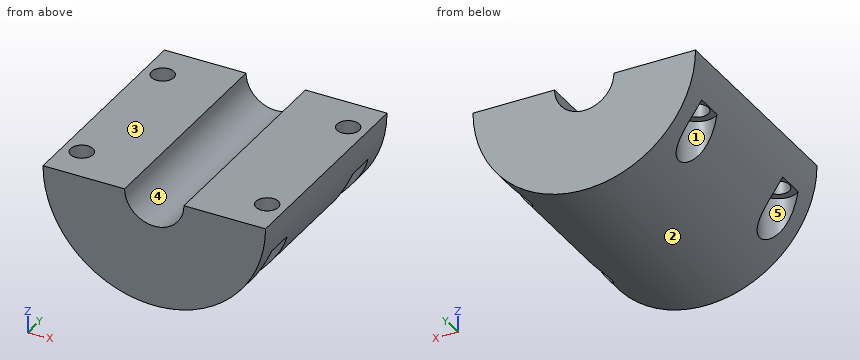
Solid Edge part; units mm, degrees
sketch "Sketch1" plane through (0, 0, 0) normal (0, -1, 0) x (1, 0, 0)
  line L0 (4, 0) -> (15, 0)
  line L1 (-15, 0) -> (-4, 0)
  arc A0 (-4, 0) -> (4, 0) centre (0, 0) ccw
  arc A1 (15, 0) -> (-15, 0) centre (0, 0) cw
extrude "Protrusion1" add sketch "Sketch1" against normal blind 30
sketch "Sketch2" plane through (-9.5, 15, 0) normal (0, 0, 1) x (1, 0, 0)
  circle A0 centre (-3, 10) radius 1.5
  circle A1 centre (22, 10) radius 1.5
  circle A2 centre (22, -10) radius 1.5
  circle A3 centre (-3, -10) radius 1.5
extrude "ExtrudedCutout_1" cut sketch "Sketch2" against normal blind 20
sketch "Sketch3" plane through (9.5, 15, -10) normal (0, 0, 1) x (0, -1, 0)
  circle A0 centre (-10, 3) radius 2.5
  circle A1 centre (10, 3) radius 2.5
  circle A2 centre (-10, -22) radius 2.5
  circle A3 centre (10, -22) radius 2.5
extrude "ExtrudedCutout_2" cut sketch "Sketch3" along normal mid plane 10
For this review, take the finished solid that the model builds, in its own axes (mm). Face numbers are marked on the shaded views. A direction names the side the tool comes from. Round coordinates to 2 decimals unless told otherwise and drop trailing zeros. Loops run counter-clockwise (first coordinate to the right, second up) from the corner with the lowest first, then second, coordinate; pieces in that order, holes last. Notation, with made-up numbers: (15.25, 6) - (63.25, 6) arc R18 ccw to (63.25, 11) - close; hole circle Ø8 at (-17.5, 86.25). An arc over 180 degrees is marked (long way). One line per item, written item: value. Start each with the question number.
Item 1: Take a section at B-B (x = 13.5). Give the boundary of the cut face in (y, z).
Item 2: Take a section at C-C (z = -7.5). Give the boundary of the cut face in (x, y), plus the area to 3 significant figures.
Item 3: Take a section at A-A (y = 25). Give the boundary of the cut face in (x, z).
Item 4: For the marked faces 4 and 5, list the 3-axis set-ups (+Z, -Z, +X, -X, +Y, -Y) from which the entire face can be reached by the end or side of a thin tool; tool diameter is ignored.
Item 5: The part is to be moulded in two halves that separate along X. For the marked faces 1, 2 and 3, say which applies: +X half, -X half, draft (parallel to the pull), parting line (faces both ways), or undercut.
Item 6: Clearance check with flat-ended pins moving along their axes: pin 1 Ø6 at (x, y) = (4.5, 20) entering from -Z; pin 2 Ø6 at (x, y) = (-12.5, 5) entering from -Z; pin 3 Ø4 at (y, z) = (14, -10.5) entering from -X. State where each tip first meets the part, or that it passes through.
Item 7: Take a section at D-D (y = 4). Give the boundary of the cut face in (x, z).
Item 8: For L1, parallel to Y at x = 12.5, z = -3.15; L2, parallel to Y at x = 12.5, z = -7.5; L3, parallel to Z at x = -11, y = 6, list the stretches that pass through material, from the lowest coordinate up.
Answer below:
1. outline: (0, -6.54) - (2.71, -6.54) - (2.71, -5) - (3.88, -5) - (3.88, 0) - (0, 0) - close; (6.12, -5) - (7.29, -5) - (7.29, -6.54) - (22.71, -6.54) - (22.71, -5) - (23.88, -5) - (23.88, 0) - (6.12, 0) - close; (26.12, -5) - (27.29, -5) - (27.29, -6.54) - (30, -6.54) - (30, 0) - (26.12, 0) - close
2. outline: (-12.99, 0) - (12.99, 0) - (12.99, 2.55) arc R2.5 cw (long way) to (12.99, 7.45) - (12.99, 22.55) arc R2.5 cw (long way) to (12.99, 27.45) - (12.99, 30) - (-12.99, 30) - (-12.99, 27.45) arc R2.5 cw (long way) to (-12.99, 22.55) - (-12.99, 7.45) arc R2.5 cw (long way) to (-12.99, 2.55) - close
2. area: 730 mm2
3. outline: (-15, 0) arc R15 ccw to (-14.14, -5) - (-14, -5) - (-14, 0) - close; (-11, -5) - (-10, -5) - (-10, -11.18) arc R15 ccw to (10, -11.18) - (10, -5) - (11, -5) - (11, 0) - (4, 0) arc R4 cw to (-4, 0) - (-11, 0) - close; (14, -5) - (14.14, -5) arc R15 ccw to (15, 0) - (14, 0) - close
4. face 4: +Z, +Y, -Y
4. face 5: -Z
5. face 1: undercut
5. face 2: parting line
5. face 3: draft
6. pin 1: stops at z = -14.92
6. pin 2: stops at z = -11.61
6. pin 3: stops at x = -12.36
7. outline: (-15, 0) arc R15 ccw to (-14.14, -5) - (-13.62, -5) - (-13.62, 0) - close; (-11.38, -5) - (-10.21, -5) - (-10.21, -10.99) arc R15 ccw to (10.21, -10.99) - (10.21, -5) - (11.38, -5) - (11.38, 0) - (4, 0) arc R4 cw to (-4, 0) - (-11.38, 0) - close; (13.62, -5) - (14.14, -5) arc R15 ccw to (15, 0) - (13.62, 0) - close
8. L1: y = 0 to 3.5, 6.5 to 23.5, 26.5 to 30
8. L2: y = 0 to 2.5, 7.5 to 22.5, 27.5 to 30
8. L3: z = -5 to 0
